Could you check a few things on this model? Use its own coordinates, in mm. A direction names the side the tool comes from. Coordinates: 2 decimals unless noted, no trailing zeros. Loops run counter-clockwise (first coordinate to the right, second up) from the corner with the lowest first, then second, coordinate; pieces in that order, holes last. Notation, with made-up numbers: M 60,89.25 L 74,89.25 A15 ccw 74,116.25 Z; hole C -38,45 d7. An arc over 180 degrees is marked long. Write each question's results on one line, items separated by ' | '.
```python
from build123d import *

# Parameters (mm, degrees)
SKETCH2_R           = 5
BOSS_EXTRUDE1_DEPTH = 10
SKETCH3_R           = 10
SKETCH3_R_2         = 5
BOSS_EXTRUDE2_DEPTH = 76.2
BOSS_EXTRUDE3_START = 86.2
SKETCH2_2_R         = 5
BOSS_EXTRUDE3_DEPTH = 22
SKETCH5_R           = 65
BOSS_EXTRUDE4_DEPTH = 22
SKETCH6_R           = 55
CUT_EXTRUDE1_DEPTH  = 22
SKETCH7_R           = 80
CUT_EXTRUDE2_DEPTH  = 143.366569109


with BuildPart() as part:
    # Sketch2 → Boss-Extrude1 (new body)
    with BuildSketch(Plane.XY):
        with BuildLine():
            Line((-19.794866372, 2.857142857), (-9.897433186, 71.428571429))
            ThreePointArc((-9.897433186, 71.428571429), (0, 80), (9.897433186, 71.428571429))
            Line((9.897433186, 71.428571429), (19.794866372, 2.857142857))
            ThreePointArc((19.794866372, 2.857142857), (0, -20), (-19.794866372, 2.857142857))
        make_face()
        with Locations((0, 70)):
            Circle(SKETCH2_R, mode=Mode.SUBTRACT)
        with BuildLine():
            Line((-2.5, 9.682458366), (-2.5, 12))
            Line((-2.5, 12), (2.5, 12))
            Line((2.5, 12), (2.5, 9.682458366))
            ThreePointArc((2.5, 9.682458366), (0, -10), (-2.5, 9.682458366))
        make_face(mode=Mode.SUBTRACT)
    extrude(amount=BOSS_EXTRUDE1_DEPTH)

    # Sketch3 → Boss-Extrude2 (add)
    with BuildSketch(Plane.XY.offset(10)):
        with Locations(Location((0, 70, 0), (0, 0, 171.786789298))):
            Circle(SKETCH3_R)
        with Locations((0, 70)):
            Circle(SKETCH3_R_2, mode=Mode.SUBTRACT)
    extrude(amount=BOSS_EXTRUDE2_DEPTH)

    # Sketch2<2> → Boss-Extrude3 (add)
    with BuildSketch(Plane.XY.offset(BOSS_EXTRUDE3_START)):
        with BuildLine():
            Line((-19.794866372, 2.857142857), (-9.897433186, 71.428571429))
            ThreePointArc((-9.897433186, 71.428571429), (0, 80), (9.897433186, 71.428571429))
            Line((9.897433186, 71.428571429), (19.794866372, 2.857142857))
            ThreePointArc((19.794866372, 2.857142857), (0, -20), (-19.794866372, 2.857142857))
        make_face()
        with Locations((0, 70)):
            Circle(SKETCH2_2_R, mode=Mode.SUBTRACT)
        with BuildLine():
            Line((-2.5, 9.682458366), (-2.5, 12))
            Line((-2.5, 12), (2.5, 12))
            Line((2.5, 12), (2.5, 9.682458366))
            ThreePointArc((2.5, 9.682458366), (0, -10), (-2.5, 9.682458366))
        make_face(mode=Mode.SUBTRACT)
    extrude(amount=BOSS_EXTRUDE3_DEPTH)

    # Sketch5 → Boss-Extrude4 (add)
    with BuildSketch(Plane.XY.offset(108.2)):
        Circle(SKETCH5_R)
    extrude(amount=-BOSS_EXTRUDE4_DEPTH)

    # Sketch6 → Cut-Extrude1 (cut)
    with BuildSketch(Plane.XY.offset(108.2)):
        Circle(SKETCH6_R)
    extrude(amount=-CUT_EXTRUDE1_DEPTH, mode=Mode.SUBTRACT)

    # Sketch7 → Cut-Extrude2 (cut, through all)
    with BuildSketch(Plane.XY.offset(10)):
        Circle(SKETCH7_R)
    extrude(amount=CUT_EXTRUDE2_DEPTH, mode=Mode.SUBTRACT)


solid = part.part
```
(1) Please list where these lines run through material, in increasing order: probe 1 along Y at (x, z) = (0, 2.5); probe 2 along X at (y, z) = (0, 7); probe 3 along Y at (x, z) = (1, 9). Write a range as from..to.
Reported:
probe 1: y = -20..-10, 12..65, 75..80 | probe 2: x = -20..-10, 10..20 | probe 3: y = -19.97..-9.95, 12..65.1, 74.9..79.95
(2) Which directions (+Z, -Z, +X, -X, +Y, -Y) give clear straight access to the entire face, cutting with the end or side of a thin tool? Please do faces 4 (the flat face through (14.777, 37.623, 4.93)), 5 (the flat face through (0, 12, 5)).
Reported:
face 4: +Z, -Z, +X, +Y | face 5: +Z, -Z
(3) If we mould it in two halves opening along X, with no side actions, what happens to faces 1 (the flat face through (-2.5, 11, 5)), 2 (the flat face through (-14.915, 36.663, 4.93)), 3 (the cylindrical face through (0, -20, 5))? For each: released by +X, released by -X, zero draft, split by the parting line, or undercut.
Reported:
face 1: undercut | face 2: released by -X | face 3: split by the parting line
(4) Will these pins go through, and if not, where does the flat tip stop? P1, Ø3, axis at x = 14.5, y = 17.5, coming from the -Z side; P2, Ø1.9, axis at y = 10.5, z = 3, coming from the -X side; P3, Ø4, axis at y = 52, z = 8, coming from the +X side; P4, Ø12, axis at x = 0, y = 0, coming from the +Z side.
Reported:
P1: stops at z = 0 | P2: stops at x = -18.83 | P3: stops at x = 12.99 | P4: passes through
(5) Imagine slicing it at D-D, the plane x = -8.5. List the corners of the cut face in (y, z) for me.
Reported:
outline: M -18.1,0 L -5.27,0 L -5.27,10 L -18.1,10 Z; M 5.27,0 L 75.27,0 L 75.27,10 L 5.27,10 Z
(6) Imagine slicing it at B-B, the plane x = 0. List the corners of the cut face in (y, z) for me, and give its area (3 significant figures).
Reported:
outline: M -20,0 L -10,0 L -10,10 L -20,10 Z; M 12,0 L 65,0 L 65,10 L 12,10 Z; M 75,0 L 80,0 L 80,10 L 75,10 Z | area: 680 mm2
(7) Imagine slicing it at A-A, the plane y = 0. List the corners of the cut face in (x, z) for me, and give its area (3 significant figures).
Reported:
outline: M -20,0 L -10,0 L -10,10 L -20,10 Z; M 10,0 L 20,0 L 20,10 L 10,10 Z | area: 200 mm2
(8) Imagine slicing it at C-C, the plane z = 3.25. List the corners of the cut face in (x, y) for me, and give its area (3 significant figures).
Reported:
outline: M -19.79,2.86 A20 ccw long 19.79,2.86 L 9.9,71.43 A10 ccw -9.9,71.43 Z; hole C 0,70 d10; hole M -2.5,9.68 A10 ccw long 2.5,9.68 L 2.5,12 L -2.5,12 Z | area: 2,500 mm2
